```python
from build123d import *

# Parameters (mm, degrees)
CROQUIS1_W              = 140
CROQUIS1_H              = 40
SALIENTE_EXTRUIR1_DEPTH = 3
CHAFL_N1_SIZE           = 0.5
CROQUIS4_W              = 40
CROQUIS4_H              = 5
SALIENTE_EXTRUIR3_DEPTH = 18
CHAFL_N2_SIZE           = 1.5
REDONDEO1_R             = 2
CROQUIS5_R              = 2.15
CORTAR_EXTRUIR1_DEPTH   = 4.3
CROQUIS6_W              = 35.4
CROQUIS6_H              = 35.4
CORTAR_EXTRUIR3_DEPTH   = 0.3
CROQUIS7_W              = 35.4
CROQUIS7_H              = 35.4
CORTAR_EXTRUIR5_DEPTH   = 0.3
CORTAR_EXTRUIR6_DEPTH   = 0.4


with BuildPart() as part:
    # Croquis1 → Saliente-Extruir1 (new, symmetric)
    with BuildSketch(Plane.XY):
        with Locations((0, 20)):
            Rectangle(CROQUIS1_W, CROQUIS1_H)
    extrude(amount=SALIENTE_EXTRUIR1_DEPTH, both=True)

    # Chaflán1
    chafl_n1_edges = [part.edges().sort_by_distance(p)[0] for p in [
        (70, 20, 3),
        (0, 40, 3),
        (-70, 20, 3),
        (0, 40, -3),
        (70, 20, -3),
        (0, 0, -3),
        (-70, 20, -3),
        (-70, 40, 0),
        (70, 40, 0),
        (70, 0, 0),
        (-70, 0, 0),
        (0, 0, 3),
    ]]
    chamfer(chafl_n1_edges, length=CHAFL_N1_SIZE)

    # Croquis4 → Saliente-Extruir3 (add)
    with BuildSketch(Plane.XY.offset(-3)):
        with Locations((-35, 20)):
            Rectangle(CROQUIS4_W, CROQUIS4_H)
    extrude(amount=-SALIENTE_EXTRUIR3_DEPTH)

    # Chaflán2
    chafl_n2_edges = [part.edges().sort_by_distance(p)[0] for p in [
        (-55, 20, -21),
        (-35, 22.5, -21),
        (-15, 20, -21),
        (-35, 17.5, -21),
    ]]
    chamfer(chafl_n2_edges, length=CHAFL_N2_SIZE)

    # Redondeo1
    redondeo1_edges = [part.edges().sort_by_distance(p)[0] for p in [
        (-55, 20, -3),
        (-35, 17.5, -3),
        (-15, 20, -3),
        (-35, 22.5, -3),
    ]]
    fillet(redondeo1_edges, radius=REDONDEO1_R)

    # Croquis5 → Cortar-Extruir1 (cut)
    with BuildSketch(Plane(origin=(0, 0, 0), x_dir=(1, 0, 0), z_dir=(0, 1, 0))):
        with Locations(Location((-50, 0, 0), (0, 0, 90))):
            Circle(CROQUIS5_R)
        with Locations(Location((0, 0, 0), (0, 0, 90))):
            Circle(CROQUIS5_R)
        with Locations(Location((50, 0, 0), (0, 0, 90))):
            Circle(CROQUIS5_R)
    extrude(amount=CORTAR_EXTRUIR1_DEPTH, mode=Mode.SUBTRACT)

    # Croquis6 → Cortar-Extruir3 (cut)
    with BuildSketch(Plane.XY.offset(3)):
        with Locations((35, 20)):
            Rectangle(CROQUIS6_W, CROQUIS6_H)
    extrude(amount=-CORTAR_EXTRUIR3_DEPTH, mode=Mode.SUBTRACT)

    # Croquis7 → Cortar-Extruir5 (cut)
    with BuildSketch(Plane.XY.offset(-3)):
        with Locations((35, 20)):
            Rectangle(CROQUIS7_W, CROQUIS7_H)
    extrude(amount=CORTAR_EXTRUIR5_DEPTH, mode=Mode.SUBTRACT)

    # Croquis8 → Cortar-Extruir6 (cut)
    with BuildSketch(Plane.XY.offset(-3)):
        Polygon((-38, 9), (-32, 9), (-35, 3), align=None)
    extrude(amount=CORTAR_EXTRUIR6_DEPTH, mode=Mode.SUBTRACT)


solid = part.part
```
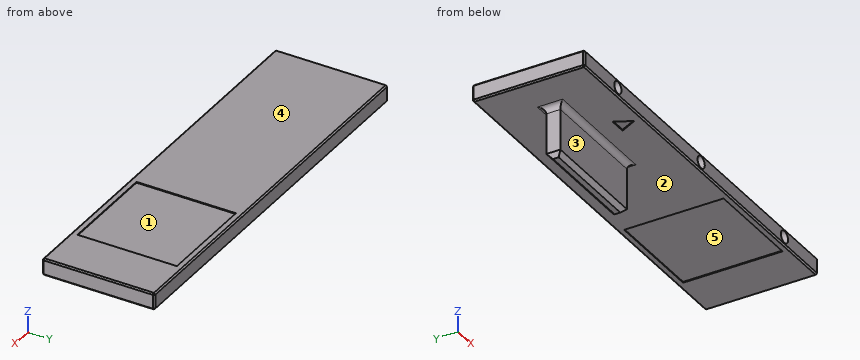
Could you check a few things on this model? Use its own coordinates, in mm. Face numbers are marked on the shaded views. A direction names the side the tool comes from. Round coordinates to 2 decimals unless told otherwise and drop trailing zeros. Loops run counter-clockwise (first coordinate to the right, second up) from the corner with the lowest first, then second, coordinate; pieces in that order, holes last. Notation, with made-up numbers: (71.5, 72) - (124.5, 72) arc R31 ccw to (124.5, 104) - close; hole circle Ø6 at (-2, -23). An arc over 180 degrees is marked (long way). Answer as CSV lines item,"result".
1. On a 3-axis mill with a long thin cutter (end or side, diameter ignored), from which of +Z, -Z, +X, -X, +Y, -Y can I reach the whole of each face in a straight line? I mean the marked faces 4 and 5. Say none if no direction works.
Filled in:
face 4,"+Z, +X, -X, +Y, -Y"
face 5,"-Z"
2. We'd pull the mould along Y, two halves only. Please class the marked faces 1, 2 and 3: +Y half, -Y half, draft (parallel to the pull), parting line (faces both ways), or undercut.
Filled in:
face 1,"undercut"
face 2,"draft"
face 3,"-Y half"
3. I want a section at D-D on x = 56. List the corners of the cut face in (y, z) for me, then the cut area to 4 significant figures.
Filled in:
outline,"(0, -2.5) - (0.5, -3) - (39.5, -3) - (40, -2.5) - (40, 2.5) - (39.5, 3) - (0.5, 3) - (0, 2.5) - close"
area,"239.5 mm^2"
4. I want a section at A-A on y = 7.5. List the corners of the cut face in (x, z) for me.
Filled in:
outline,"(-70, -2.5) - (-69.5, -3) - (-37.25, -3) - (-37.25, -2.6) - (-32.75, -2.6) - (-32.75, -3) - (17.3, -3) - (17.3, -2.7) - (52.7, -2.7) - (52.7, -3) - (69.5, -3) - (70, -2.5) - (70, 2.5) - (69.5, 3) - (52.7, 3) - (52.7, 2.7) - (17.3, 2.7) - (17.3, 3) - (-69.5, 3) - (-70, 2.5) - close"
5. For pin 1 Ø11.5 at (x, z) = (-27.5, -14.5) entering from +Y; pin 2 Ø3 at (x, y) = (48, 22) entering from -Z; pin 3 Ø4 at (y, z) = (21, -13.5) entering from +X, each with a flat end and sliding along its axis, tell me the tip position at first contact or that it passes through.
Filled in:
pin 1,"stops at y = 22.5"
pin 2,"stops at z = -2.7"
pin 3,"stops at x = -15"
6. I want a section at C-C on z = -15.25. List the corners of the cut face in (x, y) for me.
Filled in:
outline,"(-55, 17.5) - (-15, 17.5) - (-15, 22.5) - (-55, 22.5) - close"
7. Please list where these lines run through material, in increasing order: line 1 along X through (y, z) = (2.8, 0); line 2 along Z through (x, y) = (-50, 3.05); line 3 along Z through (x, y) = (-24.5, 15.5). Write a range as [from, to].
Filled in:
line 1,"x = [-70, -52.15], [-47.85, -2.15], [2.15, 47.85], [52.15, 70]"
line 2,"z = [-3, -2.15], [2.15, 3]"
line 3,"z = [-3, 3]"
8. I want a section at B-B on x = 0. List the corners of the cut face in (y, z) for me, then the cut area to 3 significant figures.
Filled in:
outline,"(0, -2.5) - (0.5, -3) - (39.5, -3) - (40, -2.5) - (40, 2.5) - (39.5, 3) - (0.5, 3) - (0, 2.5) - (0, 2.15) - (4.3, 2.15) - (4.3, -2.15) - (0, -2.15) - close"
area,"221 mm^2"
